Model file for the job. Use its own axes, mm. A direction names the side the tool comes from. Coordinates: 2 decimals unless noted, no trailing zeros. Order: outer loops, then holes, each group sorted by start corner. A loop starts at its lowest first (then second) coordinate and runs counter-clockwise, first axis right, second up. Notation, with made-up numbers: (-1, 64.25) -> (42, 64.25) arc R27 cw to (42, 95.25) -> close; hole circle Ø9 at (-20.75, -15.75). An arc over 180 degrees is marked (long way). Write item = value, one per line. Start each with the question number.
Q1. Cut at A-A, the plane z = 14.25. List the corners of the cut face in (x, y).
Q2. Flat gauge pins, fed straight in: pin 1 (1 mm diameter, centred on x = 1, y = 3.5, fed in from -Z); pin 2 (4 mm diameter, centred on y = 2.5, z = 5.5, fed in from +X); pin 3 (1.8 mm diameter, centred on x = 1, y = 0.5, fed in from +Z). Where does each tip first touch, or does it go through?
Q3. 3-axis set-ups, long thin cutter, end or side, ignore diameter. For faces 1 (the face through (-3, 0, 6)), 2 (the face through (0.74, 2.65, 14.21)), 3 (the face through (0, 0, 0)): which of +Z, -Z, +X, -X, +Y, -Y reach the whole face in a straight line?
Q4. Cut at B-B, the plane z = 8. List the corners of the cut face in (x, y), plus the area to 3 significant figures.
Q5. Wall check: line 1 (Z direction, x = -3, y = -3); line 2 (Y direction, x = 0, z = 5); line 3 (Y direction, x = 0.25, z = 12.75). Give the ranges that are in metal, low to high. Write a range as from..to.
Q6. Mould opens along Y. For faces 4 (the face through (1.93, -1.96, 14.21)), 5 (the face through (-5.357, -4.107, 12.806)), 6 (the face through (3, -1, 12)) say: +Y half, -Y half, draft (parallel to the pull), parting line (faces both ways), or undercut.
from build123d import *

# Parameters (mm, degrees)
SKETCH1_R           = 3
BOSS_EXTRUDE1_DEPTH = 12
SKETCH2_R           = 6.75
BOSS_EXTRUDE2_DEPTH = 1.5
SKETCH3_R           = 4.5
FILLET1_R           = 0.25
CUT_EXTRUDE1_DEPTH  = 2.1
CHAMFER2_SIZE       = 0.5


with BuildPart() as part:
    # Sketch1 → Boss-Extrude1 (new body)
    with BuildSketch(Plane.XY):
        Circle(SKETCH1_R)
    extrude(amount=BOSS_EXTRUDE1_DEPTH)

    # Sketch2 → Boss-Extrude2 (add)
    with BuildSketch(Plane.XY.offset(12)):
        Circle(SKETCH2_R)
    extrude(amount=BOSS_EXTRUDE2_DEPTH)

    # Sketch3 → section 1 of loft1
    with BuildSketch(Plane.XY.offset(15.25), mode=Mode.PRIVATE) as loft1_s1:
        Circle(SKETCH3_R)
    # loft up to a face of the part (loft1)
    loft([Face(Wire([part.edges().sort_by_distance((-4.620692965, 4.920538235, 13.5))[0]])), loft1_s1.sketch])

    # Fillet1
    fillet1_edges = [part.edges().sort_by_distance(p)[0] for p in [
        (-6.75, 0, 12),
        (-6.75, 0, 13.5),
        (-4.5, 0, 15.25),
    ]]
    fillet(fillet1_edges, radius=FILLET1_R)

    # Sketch6 → Cut-Extrude1 (cut)
    with BuildSketch(Plane.XY.offset(15.25)):
        Polygon((3.066485121, -0.824622541), (2.24738663, 2.243342745), (-0.819098491, 3.067965286), (-3.066485121, 0.824622541), (-2.24738663, -2.243342745), (0.819098491, -3.067965286), align=None)
    extrude(amount=-CUT_EXTRUDE1_DEPTH, mode=Mode.SUBTRACT)

    # Chamfer2
    chamfer2_edges = [part.edges().sort_by_distance(p)[0] for p in [
        (-3, 0, 0),
    ]]
    chamfer(chamfer2_edges, length=CHAMFER2_SIZE)


solid = part.part
Here are the results:
q1.outline = circle Ø11.57 at (0, 0); hole (-3.07, 0.82) -> (-2.25, -2.24) -> (0.82, -3.07) -> (3.07, -0.82) -> (2.25, 2.24) -> (-0.82, 3.07) -> close
q2.pin_1 = 12
q2.pin_2 = 2.96
q2.pin_3 = 13.15
q3.face_1 = -Z
q3.face_2 = +Z
q3.face_3 = -Z, +X, -X, +Y, -Y
q4.outline = circle Ø6 at (0, 0)
q4.area = 28.3 mm²
q5.line_1 = 12..15.25
q5.line_2 = -3..3
q5.line_3 = -6.75..6.75
q6.face_4 = undercut
q6.face_5 = parting line
q6.face_6 = draft
